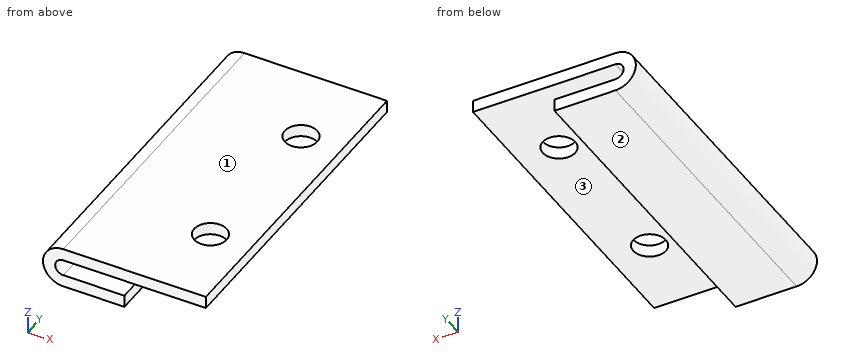
from build123d import *

# Parameters (mm, degrees)
SKETCH_1_W             = 20
SKETCH_1_H             = 40
SKETCH_1_R             = 2
SM_BASE_FLANGE_1_DEPTH = 1.5
OTHER_START            = -20
OTHER_1_DEPTH          = 40
OTHER_1_2_DEPTH        = 40


# Read off the part's stored shape, not the designer's step: 褶边1
# Sheet-metal steps are written as plain solids
with BuildPart() as part:
    # Sketch 1 → 基体-法兰1 (new body)
    with BuildSketch(Plane.XY):
        Rectangle(SKETCH_1_W, SKETCH_1_H)
        with Locations((5, 10)):
            Circle(SKETCH_1_R, mode=Mode.SUBTRACT)
        with Locations((5, -10)):
            Circle(SKETCH_1_R, mode=Mode.SUBTRACT)
    extrude(amount=-SM_BASE_FLANGE_1_DEPTH)

    # Other 1 outline → Other 1 (cut)
    with BuildSketch(Plane(origin=(0, 0, 0), x_dir=(1, 0, 0), z_dir=(0, 1, 0)).offset(OTHER_START)):
        with BuildLine():
            ThreePointArc((-7.5, 0), (-8.869306394, 0.408349934), (-9.791287847, 1.5))
            Line((-9.791287847, 1.5), (-10, 1.5))
            Line((-10, 1.5), (-10, 0))
            Line((-10, 0), (-7.5, 0))
        make_face()
    extrude(amount=OTHER_1_DEPTH, mode=Mode.SUBTRACT)

    # Other 1 2 outline → Other 1 2 (add)
    with BuildSketch(Plane(origin=(0, 0, 0), x_dir=(1, 0, 0), z_dir=(0, 1, 0)).offset(OTHER_START)):
        with BuildLine():
            Line((0, 3.5), (0, 5))
            Line((0, 5), (-7.5, 5))
            ThreePointArc((-7.5, 5), (-9.591650066, 3.869306394), (-9.791287847, 1.5))
            Line((-9.791287847, 1.5), (-7.5, 1.5))
            ThreePointArc((-7.5, 1.5), (-8.5, 2.5), (-7.5, 3.5))
            Line((-7.5, 3.5), (0, 3.5))
        make_face()
    extrude(amount=OTHER_1_2_DEPTH)


solid = part.part
The listing builds one solid part. Answer for the finished solid, in the listing's coordinates (mm). Face numbers are marked on the shaded views. Give positions to 0.01 mm unless a question says otherwise; leave off trailing zeros. Write each loop counter-clockwise with the first axis right and the second up, starting at its lowest first coordinate (ties: lowest second). Pieces come first, ordered by that corner, then holes. Notation, with made-up numbers: (52, -21) -> (75, -21) arc R12 ccw to (75, -4) -> close; hole circle Ø3 at (54.5, 57). An arc over 180 degrees is marked (long way). Use a Markdown table: item, result.
(1) Section C-C, the plane x = 5 is taken. Determine the outline of the cut face in (y, z).
Return value:
| item | result |
|---|---|
| outline | (-20, -1.5) -> (-12, -1.5) -> (-12, 0) -> (-20, 0) -> close; (-8, -1.5) -> (8, -1.5) -> (8, 0) -> (-8, 0) -> close; (12, -1.5) -> (20, -1.5) -> (20, 0) -> (12, 0) -> close |
(2) Find the intervals of material crossed by probe 1 along Y at (x, z) = (5, -0.9); probe 2 along Z at (x, y) = (-0.75, -16); probe 3 along Z at (x, y) = (7.75, -16), in increasing order. Write a range as from..to.
Return value:
| item | result |
|---|---|
| probe 1 | -20..-12, -8..8, 12..20 |
| probe 2 | -5..-3.5, -1.5..0 |
| probe 3 | -1.5..0 |
(3) Section D-D, the plane y = -13 is taken. Determine the outline of the cut face in (x, z).
Return value:
| item | result |
|---|---|
| outline | (-7.5, -5) -> (0, -5) -> (0, -3.5) -> (-7.5, -3.5) arc R1 cw to (-7.5, -1.5) -> (10, -1.5) -> (10, 0) -> (-7.5, 0) arc R2.5 ccw to start |
(4) A flat-ended cylindrical pin translates along its axis: P1, Ø2, axis at y = -10.5, z = -3, coming from the +X side. Find the tip coordinate at first contact, or state that the pin passes through.
Return value:
| item | result |
|---|---|
| P1 | x = 0 |
(5) Determine the mould class of the marked faces 1, 2 and 3 for opening direction Z: released by +Z, released by -Z, zero draft, split by the parting line, or undercut.
Return value:
| item | result |
|---|---|
| face 1 | released by +Z |
| face 2 | released by -Z |
| face 3 | undercut |
(6) Section B-B, the plane y = 10 is taken. Determine the outline of the cut face in (x, z).
Return value:
| item | result |
|---|---|
| outline | (-7.5, -5) -> (0, -5) -> (0, -3.5) -> (-7.5, -3.5) arc R1 cw to (-7.5, -1.5) -> (3, -1.5) -> (3, 0) -> (-7.5, 0) arc R2.5 ccw to start; (7, -1.5) -> (10, -1.5) -> (10, 0) -> (7, 0) -> close |
(7) Section A-A, the plane x = -6.5 is taken. Determine the outline of the cut face in (y, z), then the cut area to 3 significant figures.
Return value:
| item | result |
|---|---|
| outline | (-20, -5) -> (20, -5) -> (20, -3.5) -> (-20, -3.5) -> close; (-20, -1.5) -> (20, -1.5) -> (20, 0) -> (-20, 0) -> close |
| area | 120 mm2 |
